Autodesk Inventor part; units mm, degrees
ref_plane "YZ Plane" through (0, 0, 0) normal (1, 0, 0) x (0, 1, 0)
ref_plane "XZ Plane" through (0, 0, 0) normal (0, 1, 0) x (-1, 0, 0)
ref_plane "XY Plane" through (0, 0, 0) normal (0, 0, 1) x (1, 0, 0)
sketch "スケッチ1" plane through (0, 0, 0) normal (0, 0, 1) x (1, 0, 0)
  circle A0 centre (0, 0) radius 2
  circle A1 centre (-15, 0) radius 2
  line L0 (-41.2338, 3.4977) -> (3.0825, 11.3119)
  line L1 (-18.0894, 0) -> (0, 0)
  line L2 (3.0825, 11.3119) -> (2.5616, 14.2663)
  line L3 (2.5616, 14.2663) -> (-12.2105, 11.6616)
  line L4 (-12.2105, 11.6616) -> (-11.6896, 8.7071)
  line L5 (-26.4617, 6.1024) -> (-26.9826, 9.0568)
  line L6 (-26.9826, 9.0568) -> (-41.7547, 6.4521)
  line L7 (-41.7547, 6.4521) -> (-41.2338, 3.4977)
  line L8 (-41.2338, 3.4977) -> (-40.3656, -1.4264)
  line L9 (-40.3656, -1.4264) -> (-15.9724, -7.4585)
  arc A2 (0.8682, -4.924) -> (4.924, 0.8682) centre (0, 0) ccw
  line L10 (-13.9039, -7.5288) -> (0.8682, -4.924)
  line L11 (3.0825, 11.3119) -> (4.924, 0.8682)
  line L12 (-38.2794, 4.0186) -> (-37.7584, 1.0642)
  line L13 (-37.7584, 1.0642) -> (-28.8952, 2.627)
  line L14 (-28.8952, 2.627) -> (-29.4161, 5.5815)
  line L15 (-8.7351, 9.2281) -> (-8.2142, 6.2737)
  line L16 (-8.2142, 6.2737) -> (0.6491, 7.8365)
  line L17 (0.6491, 7.8365) -> (0.1281, 10.7909)
  circle A3 centre (-37.2453, 4.201) radius 1.05
  circle A4 centre (-30.4502, 5.3991) radius 1.05
  circle A5 centre (-29.9292, 2.4447) radius 1.05
  circle A6 centre (-36.7244, 1.2465) radius 1.05
  circle A7 centre (-7.7011, 9.4104) radius 1.05
  circle A8 centre (-0.9059, 10.6086) radius 1.05
  circle A9 centre (-0.385, 7.6542) radius 1.05
  circle A10 centre (-7.1802, 6.456) radius 1.05
  circle A11 centre (-25.4276, 6.2847) radius 1.05
  circle A12 centre (-12.7236, 8.5248) radius 1.05
  arc A13 (-15.9724, -7.4585) -> (-13.9039, -7.5288) centre (-14.7721, -2.6047) ccw
  line L18 (-14.7721, -2.6047) -> (0, 0)
  circle A14 centre (-14.7721, -2.6047) radius 2
  point P0 (-11.6896, 8.7071)
  point P1 (-13.7577, 8.3425)
  point P2 (-24.3936, 6.4671)
  point P3 (-26.4617, 6.1024)
  point P4 (-6.667, 9.5927)
  point P5 (-1.94, 10.4262)
  point P6 (0.1281, 10.7909)
  point P7 (-1.419, 7.4718)
  point P8 (-6.1461, 6.6383)
  point P9 (-8.2142, 6.2737)
  point P10 (-29.4161, 5.5815)
  point P11 (-28.8952, 2.627)
  point P12 (-30.9633, 2.2624)
  point P13 (-35.6903, 1.4289)
  point P14 (-37.7584, 1.0642)
  point P15 (-38.2794, 4.0186)
  point P16 (-36.2113, 4.3833)
  point P17 (-31.4842, 5.2168)
  point P18 (-16.3939, -1.4343)
  point P19 (-13.3783, -1.1704)
  dimension "d0" = 4
  dimension "d1" = 4
  dimension "d2" = 15
  dimension "d4" = 10
  dimension "d5" = 3
  dimension "d6" = 15
  dimension "d7" = 3
  dimension "d8" = 15
  dimension "d9" = 10
  dimension "d10" = 3
  dimension "d11" = 9
  dimension "d12" = 3
  dimension "d13" = 9
  dimension "d14" = 3
  dimension "d15" = 3
  dimension "d16" = 5
  dimension "d19" = 15
  dimension "d20" = 2.1
  dimension "d21" = 2.1
  dimension "d22" = 2.1
  dimension "d23" = 2.1
  dimension "d24" = 2.1
  dimension "d25" = 2.1
  dimension "d26" = 2.1
  dimension "d27" = 2.1
  dimension "d28" = 2.1
  dimension "d29" = 2.1
  dimension "d33" = 5
  dimension "d34" = 15
  dimension "d35" = 10
  dimension "d36" = 4
  dimension "d37" = 8
extrude "押し出し1" add sketch "スケッチ1" along normal blind 3 contours A0 L18 A14 A1 L1 | L7 L6 L5 L0 A4 A3 | L0 L12 A6 L13 A5 L14 A11 A12 L15 A10 L16 A9 L17 L11 A2 L10 A13 L9 L8 | L4 L3 L2 L0 A8 A7
fillet "フィレット1" radius 2 1 edges at (-40.3656, -1.4264, 1.5)
properties part number "シールド根本"
Work out the finished part from the listing and answer in its coordinate system (mm). A direction names the side the tool comes from. Round coordinates to 2 decimals unless told otherwise and drop trailing zeros. Loops run counter-clockwise (first coordinate to the right, second up) from the corner with the lowest first, then second, coordinate; pieces in that order, holes last. Notation, with made-up numbers: M 36.25,23.25 L 91.25,23.25 A17 cw 91.25,44.25 Z; hole C 2,-27 d6. An arc over 180 degrees is marked long. Use CSV: the item, a comma, the result in double quotes.
Q1. Section B-B, the plane z = 1.7 is taken. State how many separate pieces and enclosed holes the cut face has, then the cut area to 3 significant figures.
Determined:
separate pieces,"1"
enclosed holes,"4"
area,"553 mm2"
Q2. Each of these flat-tipped pins is pushed along its axis until it touches: pin 1 (1.5 mm diameter, centred on x = -8, z = 2.5, fed in from +Y); pin 2 (1.5 mm diameter, centred on x = -6.5, z = 1, fed in from -Y). Where does it stop, or does it pass through?
Determined:
pin 1,"y = 12.54"
pin 2,"y = -6.36"
Q3. Consider L1, parallel to Y at x = -16.5, z = 1.4; L2, parallel to Y at x = -7, z = 0.95; L3, parallel to Y at x = -37.5, z = 0.25. Determine where each line is inside the solid, lowest interval first.
Determined:
L1,"-7.33 to -3.61, -1.6 to -1.32, 1.32 to 7.86"
L2,"-6.31 to 5.42, 10.19 to 12.58"
L3,"-2.14 to 0.54, 5.22 to 7.2"
Q4. Section C-C, the plane x = -33 is taken. Determine the outline of the cut face in (y, z).
Determined:
outline,"M -3.25,0 L 1.9,0 L 1.9,3 L -3.25,3 Z; M 4.95,0 L 8,0 L 8,3 L 4.95,3 Z"
Q5. A tool of negligible diameter and unlimited length cuts with its end or side. For faces 4 (the cylindrical face through (-14.927, -7.602, 1.479)), 5 (the flat face through (-19.15, 7.39, 1.48)), 6 (the flat face through (-4.337, 10.004, 1.479)), from which of +Z, -Z, +X, -X, +Y, -Y can it reach the whole face along a straight path? Write none if from no direction.
Determined:
face 4,"+Z, -Z, -Y"
face 5,"+Z, -Z, +Y"
face 6,"+Z, -Z"
Q6. The mould has two halves that part along X. Classify faces 1 (the flat face through (-26.72, 7.56, 1.48)), 2 (the cylindrical face through (4, -3, 1)), 3 (the flat face through (-27.7, -4.56, 1.48)): pulls with the +X half, pulls with the -X half, needs draft (parallel to the pull), parting line crosses it, or undercut.
Determined:
face 1,"undercut"
face 2,"pulls with the +X half"
face 3,"pulls with the -X half"
Q7. Section D-D, the plane x = -22.5 is taken. Determine the outline of the cut face in (y, z).
Determined:
outline,"M -5.84,0 L 6.8,0 L 6.8,3 L -5.84,3 Z"
Q8. Section A-A, the plane x = -15 is taken. Determine the outline of the cut face in (y, z).
Determined:
outline,"M -7.6,0 L -4.59,0 L -4.59,3 L -7.6,3 Z; M 2,0 L 8.12,0 L 8.12,3 L 2,3 Z"
